Autodesk Inventor part; units mm, degrees
ref_plane "Work Plane2" through (36.5, 0, 0) normal (1, 0, 0) x (0, 1, 0)
ref_plane "Work Plane3" through (0, 93, 0) normal (0, 1, 0) x (1, 0, 0)
ref_plane "Work Plane5" through (0, 32, 0) normal (0, 1, 0) x (1, 0, 0)
sketch "Sketch1" plane through (0, 0, 0) normal (0, 1, 0) x (-1, 0, 0)
  circle A0 centre (0, 0) radius 36.5
  circle A1 centre (0, 0) radius 35
  dimension "d0" = 73
  dimension "d1" = 70
extrude "Extrusion1" add sketch "Sketch1" along normal blind 3 contours A0 | A1
extrude "Extrusion2" add sketch "Sketch1" along normal blind 120
sketch "Sketch2" plane through (0, 3, 0) normal (0, 1, 0) x (1, 0, 0)
  circle A0 centre (0, 0) radius 35
  line L0 (-24.7487, -24.7487) -> (24.7487, -24.7487)
  line L1 (24.7487, -24.7487) -> (24.7487, 24.7487)
  line L2 (24.7487, 24.7487) -> (-24.7487, 24.7487)
  line L3 (-24.7487, 24.7487) -> (-24.7487, -24.7487)
  line L4 (-24.7487, -24.7487) -> (24.7487, 24.7487) construction
  line L5 (24.7487, -24.7487) -> (-24.7487, 24.7487) construction
extrude "Extrusion3" add sketch "Sketch2" along normal blind 2 contours L1 L0 L3 L2
sketch "Sketch3" plane through (0, 5, 0) normal (0, 1, 0) x (1, 0, 0)
  line L0 (21.1, -23.1) -> (-21.1, -23.1)
  line L1 (-23.1, -21.1) -> (-23.1, 21.1)
  line L2 (-21.1, 23.1) -> (21.1, 23.1)
  line L3 (23.1, 21.1) -> (23.1, -21.1)
  line L4 (23.1, -23.1) -> (-23.1, 23.1) construction
  line L5 (-23.1, -23.1) -> (23.1, 23.1) construction
  arc A0 (-23.1, -21.1) -> (-21.1, -23.1) centre (-21.1, -21.1) ccw
  arc A1 (21.1, -23.1) -> (23.1, -21.1) centre (21.1, -21.1) ccw
  arc A2 (23.1, 21.1) -> (21.1, 23.1) centre (21.1, 21.1) ccw
  arc A3 (-21.1, 23.1) -> (-23.1, 21.1) centre (-21.1, 21.1) ccw
  point P0 (0, 0)
  dimension "d11" = 46.2
  dimension "d12" = 46.2
  dimension "d13" = 2
extrude "Extrusion4" cut sketch "Sketch3" against normal blind 2
sketch "Sketch4" plane through (0, 0, 0) normal (1, 0, 0) x (0, 1, 0)
  line L0 (120, 35) -> (120, -35)
  line L1 (120, 0) -> (120, -19.5)
  line L2 (120, -19.5) -> (120, -27)
  circle A0 centre (120, -27) radius 9
  point P0 (0, 0)
  dimension "d16" = 19.5
  dimension "d17" = 7.5
  dimension "d18" = 18
extrude "Extrusion5" cut sketch "Sketch4" along normal through all
sketch "Sketch5" plane through (0, 0, 0) normal (0, -1, 0) x (1, 0, 0)
  line L0 (5, -36.1559) -> (5, -42.4125)
  line L1 (5, -42.4125) -> (-5, -42.4125)
  line L2 (-5, -42.4125) -> (-5, -36.1559)
  line L3 (-5, -30.5875) -> (5, -42.4125) construction
  line L4 (5, -30.5875) -> (-5, -42.4125) construction
  circle A0 centre (0, 0) radius 36.5
  line L5 (8, -35.6125) -> (8, -42.4125)
  line L6 (8, -42.4125) -> (-8, -42.4125)
  line L7 (-8, -42.4125) -> (-8, -35.6125)
  line L8 (-8, -30.5875) -> (8, -42.4125) construction
  line L9 (8, -30.5875) -> (-8, -42.4125) construction
  circle A1 centre (0, 0) radius 36.5
  arc A2 (5, -36.1675) -> (4.9876, -36.1576) centre (0, -42.4125) ccw
  arc A3 (-4.9876, -36.1576) -> (-5, -36.1675) centre (0, -42.4125) ccw
  arc A4 (-8, -42.4125) -> (8, -42.4125) centre (0, -42.4125) ccw
  arc A5 (-5, -42.4125) -> (5, -42.4125) centre (0, -42.4125) ccw
  point P0 (0, -36.5)
  dimension "d21" = 10
  dimension "d22" = 36.5
  dimension "d23" = 16
extrude "Extrusion6" add sketch "Sketch5" against normal blind 6 contours A0 L5 L6 L0 | L6 A4 A5 | L6 L7 A0 L2
ref_plane "Work Plane2" through (36.5, 0, 0) normal (1, 0, 0) x (0, 1, 0)
sketch "Sketch8" plane through (36.5, 0, 0) normal (1, 0, 0) x (0, 1, 0)
  line L0 (8.45, 4.25) -> (21.55, 4.25)
  line L1 (21.55, 4.25) -> (21.55, -4.25)
  line L2 (21.55, -4.25) -> (8.45, -4.25)
  line L3 (8.45, -4.25) -> (8.45, 4.25)
  line L4 (8.45, 4.25) -> (21.55, -4.25) construction
  line L5 (21.55, 4.25) -> (8.45, -4.25) construction
  line L6 (7.5, 5.25) -> (22.5, 5.25)
  line L7 (22.5, 5.25) -> (22.5, -5.25)
  line L8 (22.5, -5.25) -> (7.5, -5.25)
  line L9 (7.5, -5.25) -> (7.5, 5.25)
  line L10 (7.5, 5.25) -> (22.5, -5.25) construction
  line L11 (22.5, 5.25) -> (7.5, -5.25) construction
  point P0 (0, 0)
  point P1 (15, 0)
  dimension "d38" = 13.1
  dimension "d39" = 8.5
  dimension "d40" = 0
  dimension "d41" = 15
  dimension "d42" = 10.5
  dimension "d43" = 15
extrude "Extrusion9" cut sketch "Sketch8" against normal blind 3 contours L0 L1 L2 L3
extrude "Extrusion10" cut sketch "Sketch8" against normal blind 1
ref_plane "Work Plane3" through (0, 93, 0) normal (0, 1, 0) x (1, 0, 0)
ref_plane "Work Plane5" through (0, 32, 0) normal (0, 1, 0) x (1, 0, 0)
sketch "Sketch13" plane through (0, 32, 0) normal (0, 1, 0) x (1, 0, 0)
  circle A0 centre (0, 0) radius 20
  line L0 (24.7487, 24.7487) -> (-24.7487, 24.7487)
  circle A1 centre (0, 0) radius 35
  dimension "d61" = 40
extrude "Extrusion14" add sketch "Sketch13" along normal blind 3
sketch "Sketch14" plane through (0, 32, 0) normal (0, 1, 0) x (1, 0, 0)
  circle A0 centre (0, 0) radius 50.5551
extrude "Extrusion15" cut sketch "Sketch14" against normal through all
properties part number "Outside holder"
Geometry: final body of the model. Coordinates: model frame, mm. A direction names the side the tool comes from. Coordinates: 2 decimals unless noted, no trailing zeros. Order: outer loops, then holes, each group sorted by start corner. A loop starts at its lowest first (then second) coordinate and runs counter-clockwise, first axis right, second up. Notation, with made-up numbers: (77, -8) - (110, -8) arc R15 ccw to (110, 8) - close; hole circle Ø11 at (21, -24.5). An arc over 180 degrees is marked (long way). Use one line per item in the form item = value.
1) Set-up query: faces 4 (the face through (15, 35, 15)), 5 (the face through (-4.336, 33.479, -19.524)), 6 (the face through (14.626, 112.517, -32.001)). Return all of +Z, -Z, +X, -X, +Y, -Y with unobstructed straight access to the full face (end or side cutting, diameter ignored); none if empty.
Solutions:
face_4 = +Y
face_5 = +Y, -Y
face_6 = +X, +Y
2) Section B-B (x = -3). Return loops of the section in (y, z), then the cut area to 3 significant figures.
Solutions:
outline = (32, -36.38) - (120, -36.38) - (120, -34.87) - (35, -34.87) - (35, -19.77) - (32, -19.77) - close; (32, 19.77) - (35, 19.77) - (35, 34.87) - (120, 34.87) - (120, 36.38) - (32, 36.38) - close
area = 356 mm^2
3) Section A-A (z = 0). Return loops of the section in (x, y).
Solutions:
outline = (-36.5, 32) - (-20, 32) - (-20, 35) - (-35, 35) - (-35, 120) - (-36.5, 120) - close; (20, 32) - (36.5, 32) - (36.5, 120) - (35, 120) - (35, 35) - (20, 35) - close
4) Section D-D (z = 26). Return loops of the section in (x, y).
Solutions:
outline = (-25.62, 32) - (25.62, 32) - (25.62, 120) - (23.43, 120) - (23.43, 35) - (-23.43, 35) - (-23.43, 120) - (-25.62, 120) - close
5) Ray query, L1, parallel to X at y = 34.15, z = 0; L2, parallel to X at y = 92, z = 0. Return the intervals inside material, ascending.
Solutions:
L1 = -36.5 to -20, 20 to 36.5
L2 = -36.5 to -35, 35 to 36.5
6) Section C-C (y = 109.5). Return loops of the section in (x, z).
Solutions:
outline = circle Ø73 at (0, 0); hole circle Ø70 at (0, 0)
7) Pin query (flat end, axial travel): pin 1 (1.5 mm diameter, centred on y = 46, z = 6.5, fed in from -X); pin 2 (1.5 mm diameter, centred on x = 16.5, y = 53, fed in from -Z); pin 3 (3 mm diameter, centred on x = 8, y = 89, fed in from +Z). Return the tip coordinate at first contact, or that it passes through.
Solutions:
pin_1 = -36.04
pin_2 = -32.93
pin_3 = 35.92
8) Mould query, pull axis Z, two halves, no side actions, for faces 1 (the face through (-16.15, 76.9, 31.05)), 2 (the face through (16, 32, 16)), 3 (the face through (-33.717, 75.384, 13.98)). Classes: +Z half, -Z half, draft (parallel to the pull), parting line (faces both ways), or undercut.
Solutions:
face_1 = undercut
face_2 = draft
face_3 = parting line
